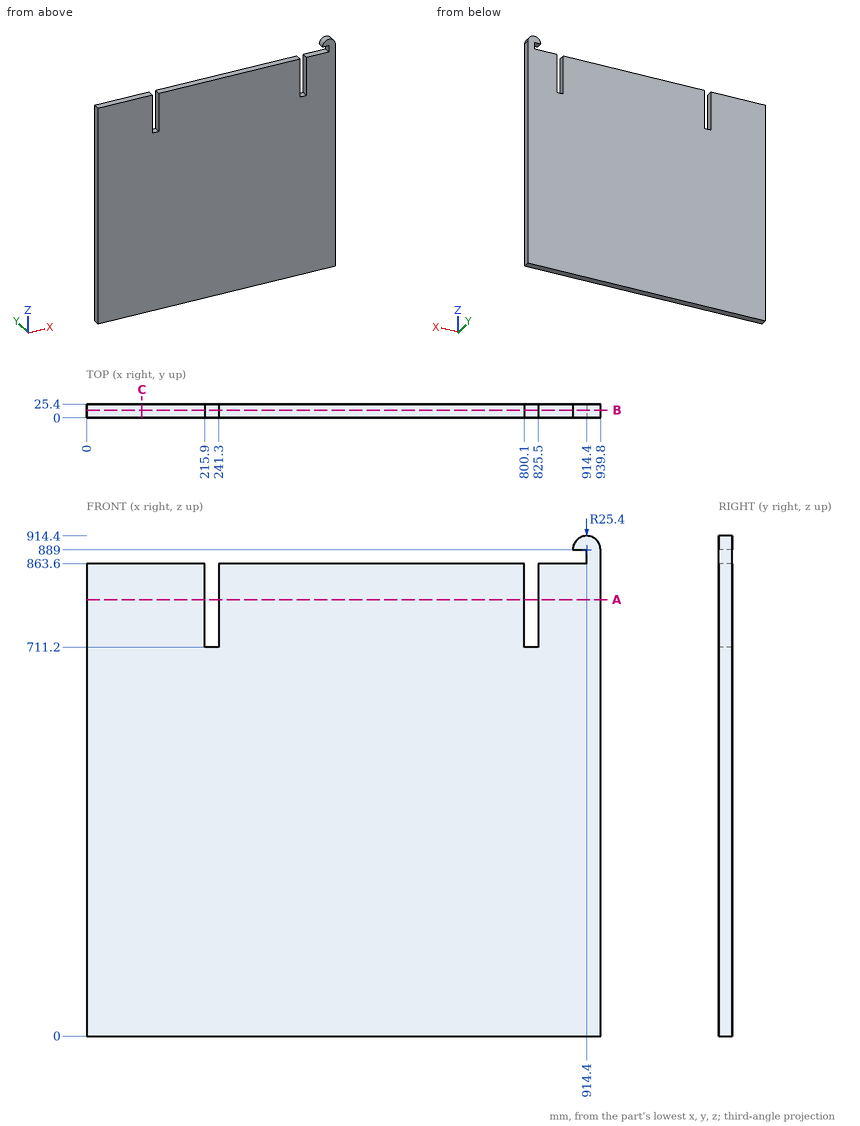
Input: dimensioned drawing with shaded views. Units: mm. Origin: part minimum x, y, z. Coordinates: 2 decimals unless noted, no trailing zeros. Order: outer loops, then holes, each group sorted by start corner. A loop starts at its lowest first (then second) coordinate and runs counter-clockwise, first axis right, second up.
1. Cut plane A-A, the plane z = 798. Return loops of the section in (x, y).
Checked values:
outline: (0, 0) - (215.9, 0) - (215.9, 25.4) - (0, 25.4) - close; (241.3, 0) - (800.1, 0) - (800.1, 25.4) - (241.3, 25.4) - close; (825.5, 0) - (939.8, 0) - (939.8, 25.4) - (825.5, 25.4) - close
2. Cut plane B-B, the plane y = 14.25. Return loops of the section in (x, z).
Checked values:
outline: (0, 0) - (939.8, 0) - (939.8, 889) arc R25.4 ccw to (889, 889) - (914.4, 889) - (914.4, 863.6) - (825.5, 863.6) - (825.5, 711.2) - (800.1, 711.2) - (800.1, 863.6) - (241.3, 863.6) - (241.3, 711.2) - (215.9, 711.2) - (215.9, 863.6) - (0, 863.6) - close
3. Cut plane C-C, the plane x = 101. Return loops of the section in (y, z).
Checked values:
outline: (0, 0) - (25.4, 0) - (25.4, 863.6) - (0, 863.6) - close
4. Contact query for flat-ended pins moving along their axis: P1, Ø1, axis at x = 331.5, y = 16, coming from the +Z side; P2, Ø12.5, axis at x = 892, y = 11, coming from the +Z side; P3, Ø12.5, axis at y = 10.5, z = 872, coming from the -X side. Output: stop coordinate, or through.
Checked values:
P1: stops at z = 863.6
P2: stops at z = 908.6
P3: stops at x = 914.4
5. Ray query, line 1 along X through (y, z) = (9.25, 756.5); line 2 along Z through (x, y) = (350, 1.25); line 3 along Z through (x, y) = (233, 13). Return the intervals inside material, ascending.
Checked values:
line 1: x = 0 to 215.9, 241.3 to 800.1, 825.5 to 939.8
line 2: z = 0 to 863.6
line 3: z = 0 to 711.2
